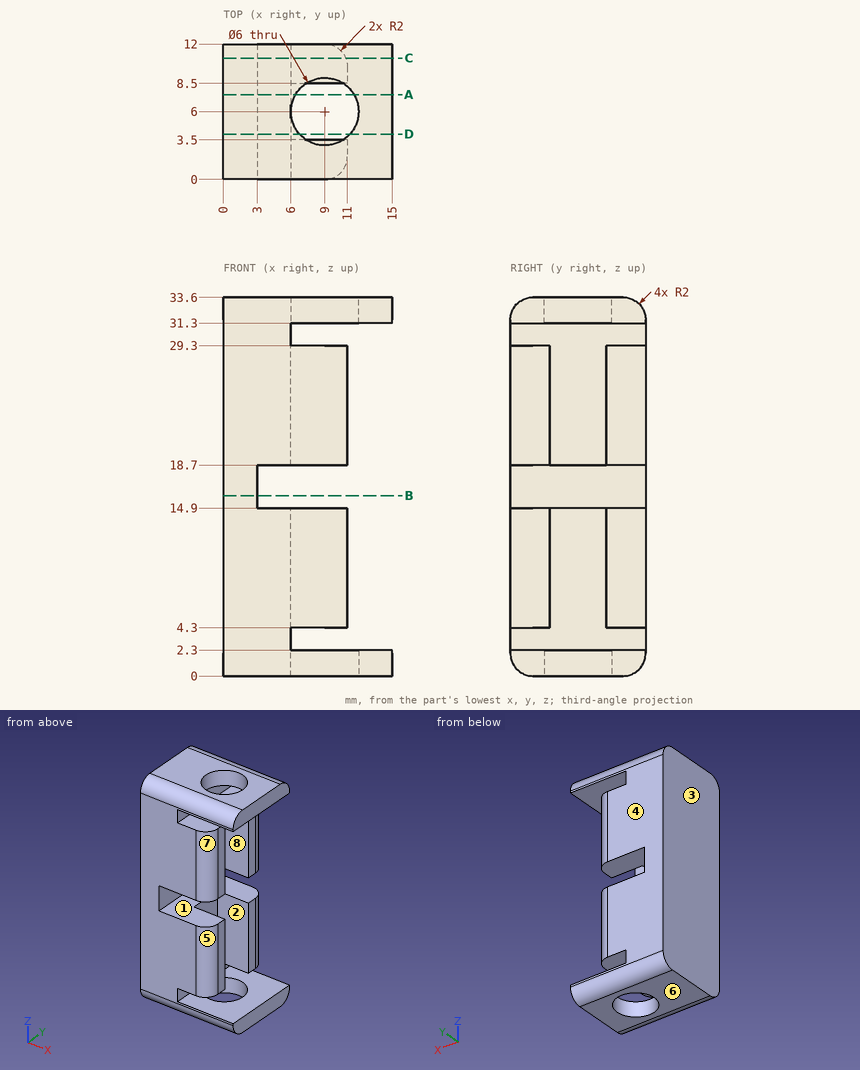
Study the drawing (mm; zero at the part's minimum x, y, z) and answer. A direction names the side the tool comes from. Coordinates: 2 decimals unless noted, no trailing zeros. Write each loop counter-clockwise with the first axis right and the second up, starting at its lowest first coordinate (ties: lowest second). Pieces come first, ordered by that corner, then holes. Notation, with made-up numbers: (21, 50.25) - (71, 50.25) arc R33 cw to (71, 78.25) - close; hole circle Ø10 at (80, 44.5). An arc over 180 degrees is marked (long way). One line per question, with ' | ' between items.
1) Flat-ended cylindrical pins translate along their axes: P1, Ø5, axis at y = 6, z = 17, coming from the +X side; P2, Ø1.2, axis at y = 9.5, z = 9, coming from the +X side; P3, Ø5.5, axis at x = 9, y = 6, coming from the -Z side. Find the tip coordinate at first contact, or state that the pin passes through.
Checks:
P1: x = 6 | P2: x = 11 | P3: z = 4.3
2) Find section B-B, the plane z = 16. Determine the outline of the cut face in (x, y), and give its area (3 significant figures).
Checks:
outline: (0, 0) - (3, 0) - (3, 12) - (0, 12) - close | area: 36.0 mm2
3) Find section D-D, the plane y = 4. Determine the outline of the cut face in (x, z).
Checks:
outline: (0, 0) - (6.76, 0) - (6.76, 2.3) - (6, 2.3) - (6, 14.9) - (3, 14.9) - (3, 18.7) - (6, 18.7) - (6, 31.3) - (6.76, 31.3) - (6.76, 33.6) - (0, 33.6) - close; (11.24, 0) - (15, 0) - (15, 2.3) - (11.24, 2.3) - close; (11.24, 31.3) - (15, 31.3) - (15, 33.6) - (11.24, 33.6) - close
4) The mould has two halves that part along Y. Classify the marked faces 6, 7 and 8: +Y half, -Y half, draft (parallel to the pull), parting line (faces both ways), or undercut.
Checks:
face 6: draft | face 7: -Y half | face 8: undercut
5) Find section C-C, the plane y = 10.75. Determine the outline of the cut face in (x, z), and give its area (3 significant figures).
Checks:
outline: (0, 0.15) - (15, 0.15) - (15, 2.3) - (6, 2.3) - (6, 4.3) - (10.85, 4.3) - (10.85, 14.9) - (3, 14.9) - (3, 18.7) - (10.85, 18.7) - (10.85, 29.3) - (6, 29.3) - (6, 31.3) - (15, 31.3) - (15, 33.45) - (0, 33.45) - close | area: 330 mm2
6) Find section A-A, the plane y = 7.5. Determine the outline of the cut face in (x, z).
Checks:
outline: (0, 0) - (6.4, 0) - (6.4, 2.3) - (6, 2.3) - (6, 14.9) - (3, 14.9) - (3, 18.7) - (6, 18.7) - (6, 31.3) - (6.4, 31.3) - (6.4, 33.6) - (0, 33.6) - close; (11.6, 0) - (15, 0) - (15, 2.3) - (11.6, 2.3) - close; (11.6, 31.3) - (15, 31.3) - (15, 33.6) - (11.6, 33.6) - close
7) Consider probe 1 along Z at (x, y) = (9.25, 2); probe 2 along Z at (x, y) = (11.75, 4.5); probe 3 along Y at (x, z) = (9.25, 27.5). Determine where each line is inside the solid, lowest interval first. Write a range as [from, to].
Checks:
probe 1: [0, 2.3], [4.3, 14.9], [18.7, 29.3], [31.3, 33.6] | probe 2: [0, 2.3], [31.3, 33.6] | probe 3: [0.02, 3.5], [8.5, 11.98]
8) For the marked faces 1, 2, 3, 4 and 5, determine the directions among +Z, -Z, +X, -X, +Y, -Y from which every point of the face is accessible in a straight line to the end or side of a thin tool.
Checks:
face 1: +X, +Y, -Y | face 2: +X | face 3: +Z, -Z, -X, +Y, -Y | face 4: +Z, -Z, +X, -X, +Y | face 5: +X, -Y
